from build123d import *

# Parameters (mm, degrees)
BOSS_EXTRUDE1_DEPTH           = 6.35
SKETCH2_W                     = 6.35
SKETCH2_H                     = 6.5278
BOSS_EXTRUDE2_DEPTH           = 6.35
SKETCH8_W                     = 6.35
SKETCH8_H                     = 6.1722
BOSS_EXTRUDE3_DEPTH           = 1.016
TAP_DRILL_FOR_6_32_TAP1_D     = 2.7051
TAP_DRILL_FOR_6_32_TAP1_DEPTH = 6.35
TAP_DRILL_FOR_6_32_TAP1_TIP   = 0.81269403
SKETCH12_W                    = 6.35
SKETCH12_H                    = 6.35
CUT_EXTRUDE2_DEPTH            = 0.08128
SKETCH13_W                    = 6.35
SKETCH13_H                    = 6.35
CUT_EXTRUDE3_DEPTH            = 0.08128
SKETCH14_W                    = 6.35
SKETCH14_H                    = 1.016
CUT_EXTRUDE4_DEPTH            = 0.0889
SKETCH15_W                    = 6.35
SKETCH15_H                    = 1.016
CUT_EXTRUDE5_DEPTH            = 0.0889


with BuildPart() as part:
    # Sketch1 → Boss-Extrude1 (new body)
    with BuildSketch(Plane(origin=(0, 0, 0), x_dir=(0, 0, -1), z_dir=(1, 0, 0))):
        Polygon((0, 0), (0, 25.4), (-2.032, 25.4), (-16.696696837, 0), align=None)
    extrude(amount=BOSS_EXTRUDE1_DEPTH)

    # Sketch2 → Boss-Extrude2 (add)
    with BuildSketch(Plane(origin=(0, 0, 0), x_dir=(-1, 0, 0), z_dir=(0, 0, -1))):
        with Locations((-3.175, 12.6111)):
            Rectangle(SKETCH2_W, SKETCH2_H)
    extrude(amount=BOSS_EXTRUDE2_DEPTH)

    # Sketch8 → Boss-Extrude3 (add)
    with BuildSketch(Plane(origin=(0, 7.22988181, 12.522522628), x_dir=(1, 0, 0), z_dir=(0, 0.49999999999999467, 0.8660254037844417))):
        with Locations((3.175, 3.035945256)):
            Rectangle(SKETCH8_W, SKETCH8_H)
    extrude(amount=BOSS_EXTRUDE3_DEPTH)

    # Tap Drill for #6-32 Tap1
    with Locations(Plane(origin=(0, 7.22988181, 12.522522628), x_dir=(1, 0, 0), z_dir=(0, 0.49999999999999467, 0.8660254037844417))):
        with Locations((3.175, 10.821045256)):
            Hole(TAP_DRILL_FOR_6_32_TAP1_D / 2, depth=TAP_DRILL_FOR_6_32_TAP1_DEPTH)
            with Locations((0, 0, -(TAP_DRILL_FOR_6_32_TAP1_DEPTH + TAP_DRILL_FOR_6_32_TAP1_TIP / 2))):  # 118° drill point
                Cone(0, TAP_DRILL_FOR_6_32_TAP1_D / 2, TAP_DRILL_FOR_6_32_TAP1_TIP, mode=Mode.SUBTRACT)

    # Sketch12 → Cut-Extrude2 (cut)
    with BuildSketch(Plane(origin=(0, 15.875, 0), x_dir=(1, 0, 0), z_dir=(0, 1, 0))):
        with Locations((3.175, 3.175)):
            Rectangle(SKETCH12_W, SKETCH12_H)
    extrude(amount=-CUT_EXTRUDE2_DEPTH, mode=Mode.SUBTRACT)

    # Sketch13 → Cut-Extrude3 (cut)
    with BuildSketch(Plane.XZ.offset(-9.3472)):
        with Locations((3.175, -3.175)):
            Rectangle(SKETCH13_W, SKETCH13_H)
    extrude(amount=-CUT_EXTRUDE3_DEPTH, mode=Mode.SUBTRACT)

    # Sketch14 → Cut-Extrude4 (cut)
    with BuildSketch(Plane(origin=(0, 5.301846715, -3.061022628), x_dir=(1, 0, 0), z_dir=(0, 0.8660254037844417, -0.49999999999999467))):
        with Locations((3.175, -14.96776362)):
            Rectangle(SKETCH14_W, SKETCH14_H)
    extrude(amount=-CUT_EXTRUDE4_DEPTH, mode=Mode.SUBTRACT)

    # Sketch15 → Cut-Extrude5 (cut)
    with BuildSketch(Plane(origin=(0, -0.043435282, 0.025077372), x_dir=(1, 0, 0), z_dir=(0, -0.8660254037844417, 0.49999999999999467))):
        with Locations((3.175, 14.96776362)):
            Rectangle(SKETCH15_W, SKETCH15_H)
    extrude(amount=-CUT_EXTRUDE5_DEPTH, mode=Mode.SUBTRACT)


solid = part.part
Geometry check sheet. Reference: the model listing, model coordinates, mm. A direction names the side the tool comes from. Round coordinates to 2 decimals unless told otherwise and drop trailing zeros. Write each loop counter-clockwise with the first axis right and the second up, starting at its lowest first coordinate (ties: lowest second). Pieces come first, ordered by that corner, then holes.
Item 1: Material ranges on line 1 along Y through (x, z) = (5, -0.5); line 2 along Y through (x, z) = (6.25, 4.25); line 3 along Z through (x, y) = (6.25, 13.75), recorded low to high.
Determined:
line 1: y = 9.43 to 15.79
line 2: y = 0 to 21.56
line 3: z = -6.35 to 8.76
Item 2: Mould release check, pull along X, two halves, no side actions. Record for faces 6 (the face through (3, 13, -6.35)), 7 (the face through (0, 10, 3)), 8 (the face through (3.002, 13.228, 0.952)): +X half, -X half, draft (parallel to the pull), parting line (faces both ways), or undercut.
Determined:
face 6: draft
face 7: -X half
face 8: undercut
Item 3: Section check D-D (y = 4.75). Record the boundary of the cut face in (x, z), plus the area to 3 significant figures.
Determined:
outline: (0, 0) - (6.35, 0) - (6.35, 13.95) - (0, 13.95) - close
area: 88.6 mm2
Item 4: Section check B-B (z = 13). Record the boundary of the cut face in (x, y).
Determined:
outline: (0, 0) - (6.35, 0) - (6.35, 6.4) - (0, 6.4) - close; (0, 7.55) - (6.35, 7.55) - (6.35, 8.43) - (0, 8.43) - close
Item 5: Section check C-C (z = -1.25). Record the boundary of the cut face in (x, y), plus the area to 3 significant figures.
Determined:
outline: (0, 9.43) - (6.35, 9.43) - (6.35, 15.79) - (0, 15.79) - close
area: 40.4 mm2
Item 6: Section check A-A (x = 1). Record the boundary of the cut face in (y, z), plus the area to 3 significant figures.
Determined:
outline: (0, 0) - (9.43, 0) - (9.43, -6.35) - (15.79, -6.35) - (15.79, 0) - (25.4, 0) - (25.4, 2.03) - (12.45, 9.51) - (12.96, 10.39) - (7.77, 13.38) - (7.26, 12.5) - (0, 16.7) - close
area: 284 mm2
Item 7: Go/stop test with a flat-tipped pin: pin 1 Ø1.9 at (x, y) = (3.5, 23) entering from -Z. Record where the tip stops, or that it passes through.
Determined:
pin 1: stops at z = 0
Item 8: Access from +Z, -Z, +X, -X, +Y, -Y to the whole of each face (thin tool, end or side, straight path). Record for faces 1 (the face through (3, 9.428, -3)), 2 (the face through (3.131, 12.705, 9.94)), 3 (the face through (3, 15.794, -3)), 4 (the face through (3.13, 7.52, 12.95)), 5 (the face through (3, 25.4, 1)).
Determined:
face 1: -Z, +X, -X, -Y
face 2: +X, -X, +Y
face 3: -Z, +X, -X, +Y
face 4: +Z, +X, -X
face 5: +Z, -Z, +X, -X, +Y
